Read the model definition and answer for the solid it produces. Units are mm, in the model's axes. A direction names the side the tool comes from. Coordinates: 2 decimals unless noted, no trailing zeros. Write each loop counter-clockwise with the first axis right and the second up, starting at its lowest first coordinate (ties: lowest second). Pieces come first, ordered by that corner, then holes.
Item 1: Each of these flat-tipped pins is pushed along its axis until it touches: P1, Ø6.5, axis at x = 12, y = 0, coming from the -Z side; P2, Ø5, axis at x = -3, z = 7.5, coming from the -Y side; P3, Ø1.2, axis at y = -9, z = 8.5, coming from the -X side; P4, Ø4, axis at x = -13.5, z = 1.5, coming from the -Y side. Where does it stop, or does it pass through?
Item 2: Section B-B (y = 0) is taken. Give the vertices of the cut face in (x, z), then the cut area to 3 significant figures.
Item 3: Section A-A (x = 0) is taken. Give the vertices of the cut face in (y, z), then the cut area to 3 significant figures.
Item 4: Straight lines are drawn through the part: probe 1 along X at (y, z) = (1.75, 2.75); probe 2 along X at (y, z) = (1.25, 3.75); probe 3 along Y at (x, z) = (11, 8). For each, find the intervals that lie inside material, in ascending order.
Item 5: Section D-D (x = 12) is taken. Give the vertices of the cut face in (y, z), then the cut area to 3 significant figures.
Item 6: Section C-C (z = 11.25) is taken. Give the vertices of the cut face in (x, y), then the cut area to 3 significant figures.
Item 7: A tool of negligible diameter and unlimited length cuts with its end or side. For faces 4 (the face through (-17.715, 5.699, 6.084)), 5 (the face through (-12, -6, 6)), 6 (the face through (11, -6, 6)), from which of +Z, -Z, +X, -X, +Y, -Y can it reach the whole face along a straight path? Write none if from no direction.
Item 8: Determine the mould class of faces 1 (the face through (0, 6, 6)), 2 (the face through (16.096, 0.18, 5.916)), 3 (the face through (-6, -8, 7)) for opening direction X: released by +X, released by -X, zero draft, split by the parting line, or undercut.
from build123d import *

# Parameters (mm, degrees)
SKETCH1_W             = 36
SKETCH1_H             = 12
BOSS_EXTRUDE1_DEPTH   = 12
F_3_0MM_DOWEL_HOLE1_D = 8.2
BOSS_EXTRUDE2_DEPTH   = 6
FILLET2_R             = 1


with BuildPart() as part:
    # Sketch1 → Boss-Extrude1 (new body)
    with BuildSketch(Plane.XY):
        Rectangle(SKETCH1_W, SKETCH1_H)
    extrude(amount=BOSS_EXTRUDE1_DEPTH)

    # Ø3.0mm Dowel Hole1 (through all)
    with Locations(Plane.XY.offset(12)):
        with Locations((-12, 0), (12, 0), (0, 0)):
            Hole(F_3_0MM_DOWEL_HOLE1_D / 2)

    # Sketch4 → Boss-Extrude2 (add, symmetric)
    with BuildSketch(Plane.ZY):
        Polygon((12, -6), (12, -10), (0, -6), align=None)
    extrude(amount=BOSS_EXTRUDE2_DEPTH, both=True)

    # Fillet2
    fillet2_edges = [part.edges().sort_by_distance(p)[0] for p in [
        (-18, 6, 6),
        (18, 6, 6),
        (18, -6, 6),
        (-18, -6, 6),
    ]]
    fillet(fillet2_edges, radius=FILLET2_R)


solid = part.part
Established:
1. P1: passes through
1. P2: stops at y = -9.33
1. P3: stops at x = -6
1. P4: stops at y = -6
2. outline: (-18, 0) - (-16.1, 0) - (-16.1, 12) - (-18, 12) - close; (-7.9, 0) - (-4.1, 0) - (-4.1, 12) - (-7.9, 12) - close; (4.1, 0) - (7.9, 0) - (7.9, 12) - (4.1, 12) - close; (16.1, 0) - (18, 0) - (18, 12) - (16.1, 12) - close
2. area: 137 mm2
3. outline: (-10, 12) - (-6, 0) - (-4.1, 0) - (-4.1, 12) - close; (4.1, 0) - (6, 0) - (6, 12) - (4.1, 12) - close
3. area: 69.6 mm2
4. probe 1: x = -18 to -15.71, -8.29 to -3.71, 3.71 to 8.29, 15.71 to 18
4. probe 2: x = -18 to -15.9, -8.1 to -3.9, 3.9 to 8.1, 15.9 to 18
4. probe 3: y = -6 to -3.98, 3.98 to 6
5. outline: (-6, 0) - (-4.1, 0) - (-4.1, 12) - (-6, 12) - close; (4.1, 0) - (6, 0) - (6, 12) - (4.1, 12) - close
5. area: 45.6 mm2
6. outline: (-18, -5) arc R1 ccw to (-17, -6) - (-6, -6) - (-6, -9.75) - (6, -9.75) - (6, -6) - (17, -6) arc R1 ccw to (18, -5) - (18, 5) arc R1 ccw to (17, 6) - (-17, 6) arc R1 ccw to (-18, 5) - close; hole circle Ø8.2 at (-12, 0); hole circle Ø8.2 at (0, 0); hole circle Ø8.2 at (12, 0)
6. area: 318 mm2
7. face 4: +Z, -Z, -X, +Y
7. face 5: +Z, -Z, -X, -Y
7. face 6: +Z, -Z, +X, -Y
8. face 1: zero draft
8. face 2: undercut
8. face 3: released by -X
